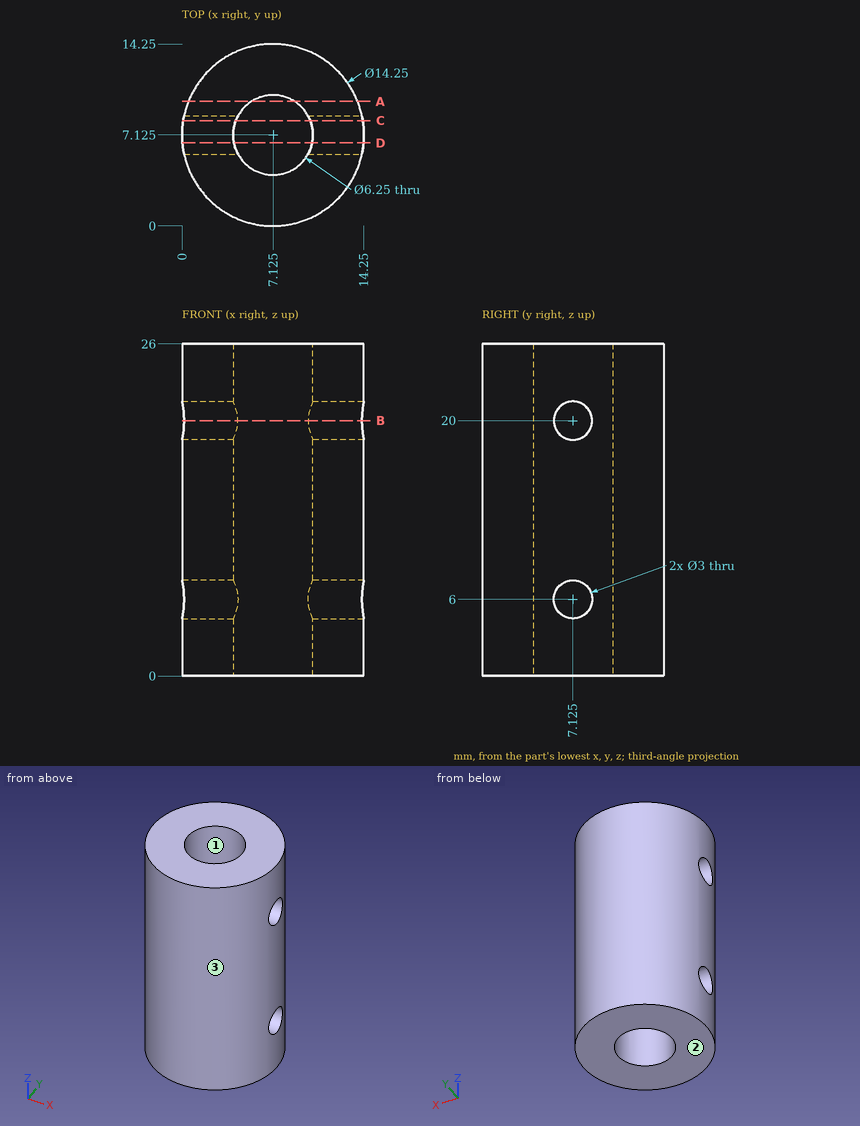
Could you check a few things on this drawing? It's one solid part, dimensions in mm from its lowest x, y, z. Round coordinates to 2 decimals unless told otherwise and drop trailing zeros. Write each loop counter-clockwise with the first axis right and the second up, starting at its lowest first coordinate (ties: lowest second). Pieces come first, ordered by that corner, then holes. Notation, with made-up numbers: M 27.25,-15.75 L 83.25,-15.75 A25 cw 83.25,12.25 Z; hole C 36,46 d6. An arc over 180 degrees is marked long. Answer as CSV lines item,"result". Start each with the question number.
1. Suppose I cut it at A-A on y = 9.75. Write out the boundary of the cut face in (x, z).
2. I need wall thicknesses on probe 1 along Y at (x, z) = (9.75, 12.5); probe 2 along X at (y, z) = (4.25, 3); probe 3 along Z at (x, y) = (11, 8.5). Which ranges of each line are inside material? Lowest first, please.
3. Suppose I cut it at B-B on z = 20. Write out the boundary of the cut face in (x, y) (3 decimals), then the cut area to 3 significant figures.
4. Suppose I cut it at D-D on y = 6.5. Write out the boundary of the cut face in (x, z).
5. Suppose I cut it at C-C on y = 8.25. Write out the boundary of the cut face in (x, z).
6. I'm going to push flat-ended pins straight in: pin 1 Ø1 at (x, z) = (1.5, 3) entering from +Y; pin 2 Ø1.5 at (x, z) = (10.5, 8) entering from -Y; pin 3 Ø4 at (x, z) = (2, 17) entering from +Y. Where does each tip first touch, or does it pass through?
7. Thinking about a two-plate mould opening in Y: for the marked faces 1, 2 and 3, which applies, released by +Y, released by -Y, zero draft, split by the parting line, or undercut?
Check result:
1,outline,"M 0.5,0 L 5.43,0 L 5.43,26 L 0.5,26 Z; M 8.82,0 L 13.75,0 L 13.75,26 L 8.82,26 Z"
2,probe 1,"y = 0.5 to 5.43, 8.82 to 13.75"
2,probe 2,"x = 0.61 to 5.9, 8.35 to 13.64"
2,probe 3,"z = 0 to 5.4, 6.6 to 19.4, 20.6 to 26"
3,outline,"M 0.16,5.625 A7.125 ccw 14.09,5.625 L 9.866,5.625 A3.125 cw 4.384,5.625 Z; M 0.16,8.625 L 4.384,8.625 A3.125 cw 9.866,8.625 L 14.09,8.625 A7.125 ccw Z"
3,area,"104 mm2"
4,outline,"M 0.03,0 L 4.06,0 L 4.06,4.64 L 0.03,4.64 Z; M 0.03,7.36 L 4.06,7.36 L 4.06,18.64 L 0.03,18.64 Z; M 0.03,21.36 L 4.06,21.36 L 4.06,26 L 0.03,26 Z; M 10.19,0 L 14.22,0 L 14.22,4.64 L 10.19,4.64 Z; M 10.19,7.36 L 14.22,7.36 L 14.22,18.64 L 10.19,18.64 Z; M 10.19,21.36 L 14.22,21.36 L 14.22,26 L 10.19,26 Z"
5,outline,"M 0.09,0 L 4.21,0 L 4.21,5.01 L 0.09,5.01 Z; M 0.09,6.99 L 4.21,6.99 L 4.21,19.01 L 0.09,19.01 Z; M 0.09,20.99 L 4.21,20.99 L 4.21,26 L 0.09,26 Z; M 10.04,0 L 14.16,0 L 14.16,5.01 L 10.04,5.01 Z; M 10.04,6.99 L 14.16,6.99 L 14.16,19.01 L 10.04,19.01 Z; M 10.04,20.99 L 14.16,20.99 L 14.16,26 L 10.04,26 Z"
6,pin 1,"stops at y = 12.07"
6,pin 2,"stops at y = 0.5"
6,pin 3,"stops at y = 13.53"
7,face 1,"undercut"
7,face 2,"zero draft"
7,face 3,"split by the parting line"
